```python
from build123d import *

# Parameters (mm, degrees)
SKETCH1_W           = 76.2
SKETCH1_H           = 101.6
BOSS_EXTRUDE1_DEPTH = 914.4
SKETCH2_W           = 63.5
SKETCH2_H           = 88.9
CUT_EXTRUDE1_DEPTH  = 917.602209249
SKETCH3_R           = 8.89
CUT_EXTRUDE2_DEPTH  = 919.974667768


with BuildPart() as part:
    # Sketch1 → Boss-Extrude1 (new body)
    with BuildSketch(Plane(origin=(0, 0, 0), x_dir=(1, 0, 0), z_dir=(0, 1, 0))):
        Rectangle(SKETCH1_W, SKETCH1_H)
    extrude(amount=BOSS_EXTRUDE1_DEPTH)

    # Sketch2 → Cut-Extrude1 (cut, through all)
    with BuildSketch(Plane(origin=(0, 914.4, 0), x_dir=(1, 0, 0), z_dir=(0, 1, 0))):
        Rectangle(SKETCH2_W, SKETCH2_H)
    extrude(amount=-CUT_EXTRUDE1_DEPTH, mode=Mode.SUBTRACT)

    # Sketch3 → Cut-Extrude2 (cut, through all)
    with BuildSketch(Plane.ZY.offset(38.1)):
        with Locations((0, 146.05)):
            Circle(SKETCH3_R)
        with Locations((0, 323.85)):
            Circle(SKETCH3_R)
    extrude(amount=-CUT_EXTRUDE2_DEPTH, mode=Mode.SUBTRACT)


solid = part.part
```
Work out the finished part from the listing and answer in its coordinate system (mm). A direction names the side the tool comes from. Give positions to 0.01 mm unless a question says otherwise; leave off trailing zeros. Order: outer loops, then holes, each group sorted by start corner. A loop starts at its lowest first (then second) coordinate and runs counter-clockwise, first axis right, second up. Notation, with made-up numbers: M 76.25,89 L 97.25,89 A19 cw 97.25,95 Z; hole C 72.5,87.5 d7. An arc over 180 degrees is marked long. Return JSON: item names as keys, results as strings.
1) Straight lines are drawn through the part: line 1 along Y through (x, z) = (-34, 0); line 2 along X through (y, z) = (784, -2.5). For each, find the intervals that lie inside material, in ascending order. Write a range as [from, to].
Resolved:
{"line 1": "[0, 137.16], [154.94, 314.96], [332.74, 914.4]", "line 2": "[-38.1, -31.75], [31.75, 38.1]"}
2) Section B-B, the plane y = 680.5 is taken. Write down the section's boundary in (x, z).
Resolved:
{"outline": "M -38.1,-50.8 L 38.1,-50.8 L 38.1,50.8 L -38.1,50.8 Z; hole M -31.75,-44.45 L 31.75,-44.45 L 31.75,44.45 L -31.75,44.45 Z"}
3) A tool of negligible diameter and unlimited length cuts with its end or side. For faces 5 (the flat face through (-31.75, 464, 1)), 6 (the flat face through (-1, 451, -50.8)), from which of +Z, -Z, +X, -X, +Y, -Y can it reach the whole face along a straight path? Write none if from no direction.
Resolved:
{"face 5": "+Y, -Y", "face 6": "-Z, +X, -X, +Y, -Y"}
4) Section A-A, the plane x = 7.5 is taken. Write down the section's boundary in (y, z), plus the area to 3 significant figures.
Resolved:
{"outline": "M 0,-50.8 L 914.4,-50.8 L 914.4,-44.45 L 0,-44.45 Z; M 0,44.45 L 914.4,44.45 L 914.4,50.8 L 0,50.8 Z", "area": "11,600 mm^2"}
5) Section D-D, the plane y = 323.85 is taken. Write down the section's boundary in (x, z), plus the area to 3 significant figures.
Resolved:
{"outline": "M -38.1,-50.8 L 38.1,-50.8 L 38.1,-8.89 L 31.75,-8.89 L 31.75,-44.45 L -31.75,-44.45 L -31.75,-8.89 L -38.1,-8.89 Z; M -38.1,8.89 L -31.75,8.89 L -31.75,44.45 L 31.75,44.45 L 31.75,8.89 L 38.1,8.89 L 38.1,50.8 L -38.1,50.8 Z", "area": "1,870 mm^2"}
6) For a pull along Y with two mould halves and no side action, classify faces 1 (the cylindrical face through (-34.969, 154.864, -1.157)), 2 (the flat face through (-34, 914.4, 0)), 3 (the cylindrical face through (34.881, 154.864, -1.157)), 4 (the flat face through (38.1, 451, 1)) as +Y half, -Y half, draft (parallel to the pull), parting line (faces both ways), or undercut.
Resolved:
{"face 1": "undercut", "face 2": "+Y half", "face 3": "undercut", "face 4": "draft"}
7) This flat-tipped pin is pushed along its axis until it touches: pin 1 (23 mm diameter, centred on y = 323.85, z = 0, fed in from -X). Where does it stop, or does it pass through?
Resolved:
{"pin 1": "x = -38.1"}
8) Section C-C, the plane z = 29 is taken. Write down the section's boundary in (x, y).
Resolved:
{"outline": "M -38.1,0 L -31.75,0 L -31.75,914.4 L -38.1,914.4 Z; M 31.75,0 L 38.1,0 L 38.1,914.4 L 31.75,914.4 Z"}
